Input: part model. Units: mm. Frame: model coordinates. Face numbers are marked on the shaded views. A direction names the side the tool comes from. Give positions to 0.01 mm unless a question says otherwise; leave off trailing zeros. Write each loop counter-clockwise with the first axis right and the second up, starting at its lowest first coordinate (ties: lowest second). Pieces come first, ordered by that corner, then holes. Notation, with made-up numbers: (-3.5, 51.25) -> (11.5, 51.25) arc R19 ccw to (11.5, 81.25) -> close; hole circle Ø5 at (-14.5, 3). An arc over 180 degrees is marked (long way). Answer as a JSON object with one key per item and string values. Group by question number.
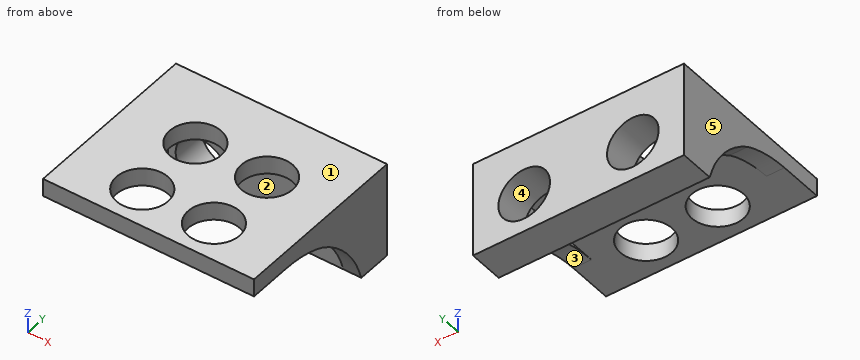
from build123d import *

# Parameters (mm, degrees)
SKETCH1_W           = 18.6944
SKETCH1_H           = 6.9088
BOSS_EXTRUDE1_DEPTH = 3.0734
SKETCH2_R           = 2.286
CUT_EXTRUDE1_DEPTH  = 3.0734
SKETCH3_W           = 18.6944
SKETCH3_H           = 15.893108249
SKETCH3_R           = 2.286
BOSS_EXTRUDE3_DEPTH = 1.5875
BOSS_EXTRUDE4_DEPTH = 1.5875
BOSS_EXTRUDE5_DEPTH = 1.5875
FILLET1_R           = 10


with BuildPart() as part:
    # Sketch1 → Boss-Extrude1 (new body)
    with BuildSketch(Plane(origin=(0, 0, 0), x_dir=(1, 0, 0), z_dir=(0, 1, 0))):
        with Locations((9.3472, -3.4544)):
            Rectangle(SKETCH1_W, SKETCH1_H)
    extrude(amount=BOSS_EXTRUDE1_DEPTH)

    # Sketch2 → Cut-Extrude1 (cut)
    with BuildSketch(Plane(origin=(0, 3.0734, 0), x_dir=(1, 0, 0), z_dir=(0, 1, 0))):
        with Locations(Location((4.5339, -3.4544, 0), (0, 0, 270))):
            Circle(SKETCH2_R)
        with Locations(Location((14.1605, -3.4544, 0), (0, 0, 270))):
            Circle(SKETCH2_R)
    extrude(amount=-CUT_EXTRUDE1_DEPTH, mode=Mode.SUBTRACT)

    # Sketch3 → Boss-Extrude3 (add)
    with BuildSketch(Plane.XY.offset(6.9088)):
        with Locations((9.3472, -4.873154125)):
            Rectangle(SKETCH3_W, SKETCH3_H)
        with Locations((12.7, -9.525)):
            Circle(SKETCH3_R, mode=Mode.SUBTRACT)
        with Locations((6.35, -9.525)):
            Circle(SKETCH3_R, mode=Mode.SUBTRACT)
        with Locations((12.7, -3.175)):
            Circle(SKETCH3_R, mode=Mode.SUBTRACT)
        with Locations((6.35, -3.175)):
            Circle(SKETCH3_R, mode=Mode.SUBTRACT)
    extrude(amount=BOSS_EXTRUDE3_DEPTH)

    # Sketch4 → Boss-Extrude4 (add)
    with BuildSketch(Plane.ZY):
        Polygon((3.4544, 0), (6.9088, -6.409854124), (6.9088, 0), align=None)
    extrude(amount=-BOSS_EXTRUDE4_DEPTH)

    # Sketch5 → Boss-Extrude5 (add)
    with BuildSketch(Plane(origin=(18.6944, 0, 0), x_dir=(0, 0, -1), z_dir=(1, 0, 0))):
        Polygon((-3.4544, 0), (-6.9088, -6.409854124), (-6.9088, 0), align=None)
    extrude(amount=-BOSS_EXTRUDE5_DEPTH)

    # Fillet1
    # the kernel refuses this fillet: 10 mm, written as the material it adds along each edge
    with BuildSketch(Plane(origin=(0, -6.409854124, 6.9088), x_dir=(0, 0.8803024942448967, -0.4744128145678757), z_dir=(1, 0, 0)), Plane(origin=(18.6944, -6.409854124, 6.9088), x_dir=(0, -1, 0), z_dir=(-1, 0, 0))) as fillet1_piece_1:
        with BuildLine():
            CenterArc((FILLET1_R * 0.252306645351, -FILLET1_R), FILLET1_R, 90, 28.321125328)
            Line((-FILLET1_R * 0.222106169217, -FILLET1_R * 0.119697505755), (-FILLET1_R * 0.231594425508, -FILLET1_R * 0.10209145587))
            Line((-FILLET1_R * 0.231594425508, -FILLET1_R * 0.10209145587), (-FILLET1_R * 0.00504613290702, FILLET1_R * 0.02))
            Line((-FILLET1_R * 0.00504613290702, FILLET1_R * 0.02), (FILLET1_R * 0.252306645351, FILLET1_R * 0.02))
            Line((FILLET1_R * 0.252306645351, FILLET1_R * 0.02), (FILLET1_R * 0.252306645351, 0))
        make_face()
    extrude(amount=1.5875)
    with BuildSketch(Plane(origin=(0, 0, 3.4544), x_dir=(0, 0, -1), z_dir=(1, 0, 0))) as fillet1_piece_2:
        with BuildLine():
            CenterArc((6.173594354, -9.623200199), FILLET1_R, 105.778516421, 45.90035825)
            Line((-2.629430588, -4.879072053), (-2.805491087, -4.78418949))
            Line((-2.805491087, -4.78418949), (-0.176060499, 0.094882563))
            Line((-0.176060499, 0.094882563), (0, 0.2))
            ThreePointArc((0, 0.2), (1.7272, 0.2), (3.400016113, 0.192464004))
            Line((3.400016113, 0.192464004), (3.4544, 0))
        make_face()
    extrude(amount=1.5875)
    with BuildSketch(Plane(origin=(18.6944, 0, 3.4544), x_dir=(0, 0, -1), z_dir=(-1, 0, 0))) as fillet1_piece_3:
        with BuildLine():
            CenterArc((6.173594354, 9.623200199), FILLET1_R, 208.321125328, 45.90035825)
            Line((-2.629430588, 4.879072053), (-2.805491087, 4.78418949))
            Line((-2.805491087, 4.78418949), (-0.176060499, -0.094882563))
            Line((-0.176060499, -0.094882563), (0, -0.2))
            ThreePointArc((0, -0.2), (1.7272, -0.2), (3.400016113, -0.192464004))
            Line((3.400016113, -0.192464004), (3.4544, 0))
        make_face()
    extrude(amount=1.5875)


solid = part.part
1. Section B-B (y = -11). Return the cut outline in (x, z), plus the area to 3 significant figures.
2. Section A-A (x = 3.5). Return the cut outline in (y, z).
3. Contact query for flat-ended pins moving along their axis: pin 1 Ø4 at (x, y) = (16.5, -5.5) entering from -Z; pin 2 Ø4 at (x, y) = (12, -6) entering from -Z; pin 3 Ø1 at (x, z) = (3, 5.5) entering from -Y. Output: stop coordinate, or through.
4. Line query: line 1 (Y direction, x = 6.35, z = 7.55); line 2 (X direction, y = 1, z = 4.5); line 3 (X direction, y = 2, z = 5). Output: solid intervals per line, ascending.
5. Mould query, pull axis X, two halves, no side actions, for the marked faces 3, 4 and 5. Classes: pulls with the +X half, pulls with the -X half, needs draft (parallel to the pull), parting line crosses it, or undercut.
6. Section C-C (z = 5.25). Return the cut outline in (x, y).
7. Section D-D (x = 1). Return the cut outline in (y, z).
8. Reachability of the marked faces 1 and 2 from +Z, -Z, +X, -X, +Y, -Y: full face, straight path, thin tool, end or side. Return the list, or none.
Working result:
{
 "1": {"outline": "(0, 6.91) -> (4.6, 6.91) -> (4.6, 8.5) -> (0, 8.5) -> close; (8.1, 6.91) -> (10.95, 6.91) -> (10.95, 8.5) -> (8.1, 8.5) -> close; (14.45, 6.91) -> (18.69, 6.91) -> (18.69, 8.5) -> (14.45, 8.5) -> close", "area": "18.6 mm^2"},
 "2": {"outline": "(-12.82, 6.91) -> (0, 6.91) -> (0, 5.49) -> (3.07, 5.49) -> (3.07, 8.5) -> (-12.82, 8.5) -> close; (0, 0) -> (3.07, 0) -> (3.07, 1.42) -> (0, 1.42) -> close"},
 "3": {"pin 1": "stops at z = 5.26", "pin 2": "stops at z = 6.91", "pin 3": "stops at y = 0"},
 "4": {"line 1": "y = -12.82 to -11.81, -7.24 to -5.46, -0.89 to 3.07", "line 2": "x = 0 to 2.5, 6.57 to 12.13, 16.19 to 18.69", "line 3": "x = 0 to 2.85, 6.22 to 12.48, 15.84 to 18.69"},
 "5": {"face 3": "needs draft", "face 4": "undercut", "face 5": "pulls with the -X half"},
 "6": {"outline": "(0, -3.58) -> (1.59, -3.58) -> (1.59, 0) -> (3.12, 0) -> (3.12, 3.07) -> (0, 3.07) -> close; (5.95, 0) -> (12.75, 0) -> (12.75, 3.07) -> (5.95, 3.07) -> close; (15.58, 0) -> (17.11, 0) -> (17.11, -3.58) -> (18.69, -3.58) -> (18.69, 3.07) -> (15.58, 3.07) -> close"},
 "7": {"outline": "(-12.82, 6.91) -> (-8.93, 6.91) arc R10 cw to (-4.54, 5.89) arc R10 cw to (0, 0) -> (3.07, 0) -> (3.07, 8.5) -> (-12.82, 8.5) -> close"},
 "8": {"face 1": "+Z, +X, -X, +Y, -Y", "face 2": "-Z, -Y"}
}
